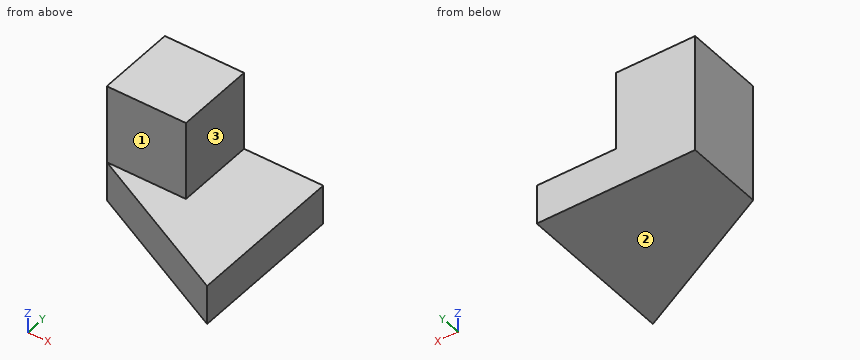
```python
from build123d import *

# Parameters (mm, degrees)
F0_W     = 1016
F0_H     = 1016
F1_DEPTH = 762
F3_DEPTH = 508
F5_DEPTH = 254


with BuildPart() as f1:
    # F0 (on Top) → F1 (new body)
    with BuildSketch(Plane.XY):
        with Locations((508, -508)):
            Rectangle(F0_W, F0_H)
    extrude(amount=F1_DEPTH)

    # F2 (on face) → F3 (cut)
    with BuildSketch(Plane.XY.offset(762)):
        Polygon((1016, 0), (508, 0), (508, -508), (0, -508), (0, -1016), (1016, -1016), align=None)
    extrude(amount=-F3_DEPTH, mode=Mode.SUBTRACT)

    # F4 (on face) → F5 (cut)
    with BuildSketch(Plane.XY.offset(254)):
        Polygon((1016, -1016), (0, -508), (0, -1016), align=None)
    extrude(amount=-F5_DEPTH, mode=Mode.SUBTRACT)


solid = f1.part
```
Can you work these out from the model? Positions are in its coordinate system, mm. Face numbers are marked on the shaded views. A direction names the side the tool comes from. Round coordinates to 2 decimals unless told otherwise and drop trailing zeros. Order: outer loops, then holes, each group sorted by start corner. A loop starts at its lowest first (then second) coordinate and runs counter-clockwise, first axis right, second up.
(1) If we section it at A-A (x = 452.5): Please give me the cut outline in (y, z).
Results are:
outline: (-734.25, 0) - (0, 0) - (0, 762) - (-508, 762) - (-508, 254) - (-734.25, 254) - close
(2) On a 3-axis mill with a long thin cutter (end or side, diameter ignored), from which of +Z, -Z, +X, -X, +Y, -Y can I reach the whole of each face in a straight line? I mean the marked faces 1, 2 and 3. Say none if no direction works.
Results are:
face 1: +Z, +X, -X, -Y
face 2: -Z, +X, -X, +Y, -Y
face 3: +Z, +X, +Y, -Y
(3) If we section it at B-B (z = 536): Please give me the cut outline in (x, y).
Results are:
outline: (0, -508) - (508, -508) - (508, 0) - (0, 0) - close
(4) If I drill on L1, parallel to X at y = -92, z = 349.5; L2, parallel to Y at x = 324.5, z = 508; L3, parallel to Z at x = 737, y = -742.5, over which ranges is the centre line in solid material (lowest first)?
Results are:
L1: x = 0 to 508
L2: y = -508 to 0
L3: z = 0 to 254
(5) If we section it at D-D (x = 908): Please give me the cut outline in (y, z), plus the area to 3 significant figures.
Results are:
outline: (-962, 0) - (0, 0) - (0, 254) - (-962, 254) - close
area: 244,000 mm2
(6) I'm going to push flat-ended pins straight in: pin 1 (5 mm diameter, centred on x = 389, y = -667.5, fed in from -Z); pin 2 (4 mm diameter, centred on y = -368, z = 365.5, fed in from +X). Where does each tip first touch, or does it pass through?
Results are:
pin 1: stops at z = 0
pin 2: stops at x = 508
(7) If we section it at C-C (y = -167): Please give me the cut outline in (x, z), plus the area to 3 significant figures.
Results are:
outline: (0, 0) - (1016, 0) - (1016, 254) - (508, 254) - (508, 762) - (0, 762) - close
area: 516,000 mm2
